Read the model definition and answer for the solid it produces. Units are mm, in the model's axes. A direction names the side the tool comes from. Round coordinates to 2 decimals unless told otherwise and drop trailing zeros. Write each loop counter-clockwise with the first axis right and the second up, starting at its lowest first coordinate (ties: lowest second). Pieces come first, ordered by that corner, then holes.
from build123d import *

# Parameters (mm, degrees)
SKETCH_1_W          = 110
SKETCH_1_H          = 60
SKETCH_1_R          = 1.5
EXTRUDE_1_DEPTH     = 3
FILLET_1_R          = 25
CHAMFER_1_SIZE      = 10
SKETCH_3_R          = 1.5
CUT_EXTRUDE_2_DEPTH = 3
SKETCH_4_W          = 13
SKETCH_4_H          = 10
CUT_EXTRUDE_3_DEPTH = 10
FILLET_2_R          = 2
SKETCH_5_R          = 1.5
SKETCH_5_R_2        = 15
CUT_EXTRUDE_4_DEPTH = 3


with BuildPart() as part:
    # 草图1 → 凸台-拉伸1 (new body)
    with BuildSketch(Plane(origin=(0, 0, 0), x_dir=(1, 0, 0), z_dir=(0, 1, 0))):
        Rectangle(SKETCH_1_W, SKETCH_1_H)
        with Locations(Location((-49, 2, 0), (0, 0, 270))):
            Circle(SKETCH_1_R, mode=Mode.SUBTRACT)
        with Locations(Location((-40, 2, 0), (0, 0, 270))):
            Circle(SKETCH_1_R, mode=Mode.SUBTRACT)
        with Locations(Location((49, 2, 0), (0, 0, 90))):
            Circle(SKETCH_1_R, mode=Mode.SUBTRACT)
        with Locations(Location((40, 2, 0), (0, 0, 90))):
            Circle(SKETCH_1_R, mode=Mode.SUBTRACT)
    extrude(amount=EXTRUDE_1_DEPTH)

    # 圆角1
    fillet_1_edges = [part.edges().sort_by_distance(p)[0] for p in [
        (-55, 1.5, -30),
        (55, 1.5, -30),
    ]]
    fillet(fillet_1_edges, radius=FILLET_1_R)

    # 倒角1
    chamfer_1_edges = [part.edges().sort_by_distance(p)[0] for p in [
        (55, 1.5, 30),
        (-55, 1.5, 30),
    ]]
    chamfer(chamfer_1_edges, length=CHAMFER_1_SIZE)

    # 草图3 → 切除-拉伸2 (cut)
    with BuildSketch(Plane(origin=(0, 3, 0), x_dir=(1, 0, 0), z_dir=(0, 1, 0))):
        with Locations(Location((-32, 19, 0), (0, 0, 270))):
            Circle(SKETCH_3_R)
        with Locations(Location((-27, -19, 0), (0, 0, 270))):
            Circle(SKETCH_3_R)
        with Locations(Location((27, -19, 0), (0, 0, 90))):
            Circle(SKETCH_3_R)
        with Locations(Location((32, 19, 0), (0, 0, 90))):
            Circle(SKETCH_3_R)
    extrude(amount=-CUT_EXTRUDE_2_DEPTH, mode=Mode.SUBTRACT)

    # 草图4 → 切除-拉伸3 (cut)
    with BuildSketch(Plane(origin=(0, 3, 0), x_dir=(1, 0, 0), z_dir=(0, 1, 0))):
        with Locations((-44.5, -13)):
            Rectangle(SKETCH_4_W, SKETCH_4_H)
        with Locations((44.5, -13)):
            Rectangle(SKETCH_4_W, SKETCH_4_H)
    extrude(amount=-CUT_EXTRUDE_3_DEPTH, mode=Mode.SUBTRACT)

    # 圆角2
    fillet_2_edges = [part.edges().sort_by_distance(p)[0] for p in [
        (-38, 1.5, 8),
        (-38, 1.5, 18),
        (-51, 1.5, 18),
        (-51, 1.5, 8),
        (51, 1.5, 8),
        (51, 1.5, 18),
        (38, 1.5, 18),
        (38, 1.5, 8),
    ]]
    fillet(fillet_2_edges, radius=FILLET_2_R)

    # 草图5 → 切除-拉伸4 (cut)
    with BuildSketch(Plane(origin=(0, 3, 0), x_dir=(1, 0, 0), z_dir=(0, 1, 0))):
        with Locations(Location((20, -4, 0), (0, 0, 270))):
            Circle(SKETCH_5_R)
        with Locations(Location((10, 13.320508076, 0), (0, 0, 270))):
            Circle(SKETCH_5_R)
        with Locations(Location((-20, -4, 0), (0, 0, 90))):
            Circle(SKETCH_5_R)
        with Locations(Location((-10, 13.320508076, 0), (0, 0, 90))):
            Circle(SKETCH_5_R)
        with Locations(Location((10, -21.320508076, 0), (0, 0, 90))):
            Circle(SKETCH_5_R)
        with Locations(Location((-10, -21.320508076, 0), (0, 0, 270))):
            Circle(SKETCH_5_R)
        with Locations(Location((0, -4, 0), (0, 0, 270))):
            Circle(SKETCH_5_R_2)
    extrude(amount=-CUT_EXTRUDE_4_DEPTH, mode=Mode.SUBTRACT)


solid = part.part
Q1. Which of the six approach directions +Z, -Z, +X, -X, +Y, -Y give full straight-line access (tool end or side, diameter ignored) to faces 1 (the flat face through (-51, 2, 13)), 2 (the flat face through (-50, 1, 25))?
Verdict:
face 1: +Y, -Y
face 2: +Z, -X, +Y, -Y
Q2. Straight lines are drawn through the part: probe 1 along X at (y, z) = (1.65, 4); probe 2 along X at (y, z) = (1.55, 21); probe 3 along Z at (x, y) = (49, 2.65). For each, find the intervals that lie inside material, in ascending order.
Verdict:
probe 1: x = -55 to -21.5, -18.5 to -15, 15 to 18.5, 21.5 to 55
probe 2: x = -54 to -11.47, -8.53 to 8.53, 11.47 to 54
probe 3: z = -21.25 to -3.5, -0.5 to 8, 18 to 26
Q3. Section A-A (x = 20) is taken. Determine the outline of the cut face in (y, z), then the cut area to 3 significant figures.
Verdict:
outline: (0, -30) - (3, -30) - (3, 2.5) - (0, 2.5) - close; (0, 5.5) - (3, 5.5) - (3, 30) - (0, 30) - close
area: 171 mm2
Q4. Section B-B (z = -2) is taken. Determine the outline of the cut face in (x, y), then the cut area to 3 significant figures.
Verdict:
outline: (-55, 0) - (-50.5, 0) - (-50.5, 3) - (-55, 3) - close; (-47.5, 0) - (-41.5, 0) - (-41.5, 3) - (-47.5, 3) - close; (-38.5, 0) - (-13.75, 0) - (-13.75, 3) - (-38.5, 3) - close; (13.75, 0) - (38.5, 0) - (38.5, 3) - (13.75, 3) - close; (41.5, 0) - (47.5, 0) - (47.5, 3) - (41.5, 3) - close; (50.5, 0) - (55, 0) - (55, 3) - (50.5, 3) - close
area: 212 mm2
Q5. Section C-C (x = -10) is taken. Determine the outline of the cut face in (y, z), then the cut area to 3 significant figures.
Verdict:
outline: (0, -30) - (3, -30) - (3, -14.82) - (0, -14.82) - close; (0, -11.82) - (3, -11.82) - (3, -7.18) - (0, -7.18) - close; (0, 15.18) - (3, 15.18) - (3, 19.82) - (0, 19.82) - close; (0, 22.82) - (3, 22.82) - (3, 30) - (0, 30) - close
area: 94.9 mm2
Q6. Section D-D (x = -32) is taken. Determine the outline of the cut face in (y, z).
Verdict:
outline: (0, -29.92) - (3, -29.92) - (3, -20.5) - (0, -20.5) - close; (0, -17.5) - (3, -17.5) - (3, 30) - (0, 30) - close
Q7. Determine the mould class of faces 3 (the cylindrical face through (47.482, 1.521, -22.871)), 4 (the cylindrical face through (10.575, 1.521, 19.935)), 5 (the flat face through (-45, 2, 18)), 6 (the flat face through (-1, 1, 30)) for opening direction X: pulls with the +X half, pulls with the -X half, needs draft (parallel to the pull), parting line crosses it, or undercut.
Verdict:
face 3: pulls with the +X half
face 4: undercut
face 5: undercut
face 6: needs draft
Q8. Flat-ended cylindrical pins translate along their axes: pin 1 Ø0.9 at (x, y) = (44.5, 2) entering from -Z; pin 2 Ø5 at (x, z) = (-10, 21.32) entering from -Y; pin 3 Ø1 at (y, z) = (1.5, 23.5) entering from +X; pin 4 Ø1.5 at (x, y) = (-44.5, 2) entering from -Z. Find the tip coordinate at first contact, or state that the pin passes through.
Verdict:
pin 1: stops at z = -25.68
pin 2: stops at y = 0
pin 3: stops at x = 52
pin 4: stops at z = -25.88
